Autodesk Fusion 360 part; units mm, degrees
sketch "Sketch1" plane through (0, 0, 0) normal (0, 0, 1) x (1, 0, 0)
  line L0 (97.7238, 100.1373) -> (197.7238, 100.1373)
  line L1 (197.7238, 100.1373) -> (197.7238, 30.1373)
  line L2 (197.7238, 30.1373) -> (97.7238, 30.1373)
  line L3 (97.7238, 30.1373) -> (97.7238, 100.1373)
  dimension "d1" = 70
  dimension "d2" = 100
extrude "Extrude1" add sketch "Sketch1" along normal blind 20
sketch "Sketch2" plane through (0, 0, 20) normal (0, 0, 1) x (-1, 0, 0)
  line L0 (-97.7238, -30.1373) -> (-197.7238, -30.1373)
  line L1 (-197.7238, -30.1373) -> (-197.7238, -100.1373)
  line L2 (-197.7238, -100.1373) -> (-97.7238, -100.1373)
  line L3 (-97.7238, -100.1373) -> (-97.7238, -30.1373)
  line L4 (-97.7238, -77.6373) -> (-127.7238, -77.6373)
  line L5 (-127.7238, -77.6373) -> (-127.7238, -52.6373)
  line L6 (-127.7238, -52.6373) -> (-97.7238, -52.6373)
  dimension "d5" = 22.5
  dimension "d6" = 22.5
  dimension "d7" = 25
  dimension "d8" = 30
  dimension "d9" = 25
extrude "Extrude2" cut sketch "Sketch2" against normal blind 27.453 contours L3 L4 L5 L6
sketch "Sketch3" plane through (0, 0, 20) normal (0, 0, 1) x (-1, 0, 0)
  line L0 (-127.7238, -52.6373) -> (-97.7238, -52.6373)
  line L1 (-97.7238, -52.6373) -> (-97.7238, -30.1373)
  line L2 (-97.7238, -30.1373) -> (-197.7238, -30.1373)
  line L3 (-197.7238, -30.1373) -> (-197.7238, -100.1373)
  line L4 (-197.7238, -100.1373) -> (-97.7238, -100.1373)
  line L5 (-97.7238, -100.1373) -> (-97.7238, -77.6373)
  line L6 (-97.7238, -77.6373) -> (-127.7238, -77.6373)
  line L7 (-127.7238, -77.6373) -> (-127.7238, -52.6373)
  line L8 (-97.7238, -52.6373) -> (-97.7238, -45.1373)
  line L9 (-97.7238, -77.6373) -> (-97.7238, -85.1373)
  line L10 (-147.7238, -30.1373) -> (-147.7238, -100.1373)
  line L11 (-97.7238, -85.1373) -> (-147.7238, -100.1373)
  line L12 (-97.7238, -45.1373) -> (-147.7238, -30.1373)
  dimension "d12" = 7.5
  dimension "d13" = 7.5
extrude "Extrude3" cut sketch "Sketch3" against normal blind 62.472 contours L1 L2 L12
extrude "Extrude4" cut sketch "Sketch3" against normal blind 73.462 contours L4 L5 L11
sketch "Sketch4" plane through (0, 30.1373, 0) normal (0, -1, 0) x (1, 0, 0)
  line L0 (147.7238, 20) -> (147.7238, 0)
  line L1 (147.7238, 0) -> (197.7238, 0)
  line L2 (197.7238, 0) -> (197.7238, 20)
  line L3 (197.7238, 20) -> (147.7238, 20)
  line L4 (197.7238, 20) -> (197.7238, 40)
  line L5 (197.7238, 40) -> (177.7238, 40)
  line L6 (177.7238, 40) -> (177.7238, 20)
  dimension "d18" = 20
  dimension "d19" = 20
extrude "Extrude5" add sketch "Sketch4" against normal blind 70 contours L3 L4 L5 L6
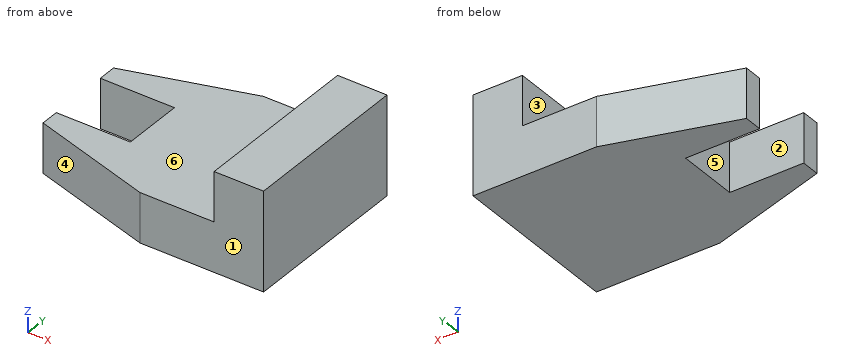
Work out the finished part from the listing and answer in its coordinate system (mm). Face numbers are marked on the shaded views. A direction names the side the tool comes from. Coordinates: 2 decimals unless noted, no trailing zeros. Loops run counter-clockwise (first coordinate to the right, second up) from the corner with the lowest first, then second, coordinate; pieces in that order, holes last.
1) Section A-A (z = 11.5) is taken. Give the vertices of the cut face in (x, y), plus the area to 3 significant figures.
Results:
outline: (97.72, 45.14) - (147.72, 30.14) - (197.72, 30.14) - (197.72, 100.14) - (147.72, 100.14) - (97.72, 85.14) - (97.72, 77.64) - (127.72, 77.64) - (127.72, 52.64) - (97.72, 52.64) - close
area: 5,500 mm2
2) Consider probe 1 along X at (y, z) = (43.5, 31); probe 2 along Z at (x, y) = (176, 73); probe 3 along X at (y, z) = (77.5, 18.5). Determine where each line is inside the solid, lowest interval first.
Results:
probe 1: x = 177.72 to 197.72
probe 2: z = 0 to 20
probe 3: x = 127.72 to 197.72
3) Flat-ended cylindrical pins translate along their axes: pin 1 (16 mm diameter, centred on x = 116, z = 9.5, fed in from +Y); pin 2 (8 mm diameter, centred on x = 139.5, z = 17.5, fed in from -Y); pin 3 (2 mm diameter, centred on x = 164, y = 48, fed in from +Z). Find the tip coordinate at first contact, or state that the pin passes through.
Results:
pin 1: stops at y = 93.02
pin 2: stops at y = 31.4
pin 3: stops at z = 20
4) For a pull along Y with two mould halves and no side action, classify the marked faces 4, 5 and 6 as +Y half, -Y half, draft (parallel to the pull), parting line (faces both ways), or undercut.
Results:
face 4: -Y half
face 5: undercut
face 6: draft
5) Section B-B (x = 106.5) is taken. Give the vertices of the cut face in (y, z), plus the area to 3 significant figures.
Results:
outline: (42.5, 0) - (52.64, 0) - (52.64, 20) - (42.5, 20) - close; (77.64, 0) - (87.77, 0) - (87.77, 20) - (77.64, 20) - close
area: 405 mm2
6) For the marked faces 1, 2 and 3, determine the directions among +Z, -Z, +X, -X, +Y, -Y from which every point of the face is accessible in a straight line to the end or side of a thin tool.
Results:
face 1: +Z, -Z, +X, -X, -Y
face 2: +Z, -Z, -X
face 3: +Z, -X, +Y, -Y
7) Section D-D (x = 175) is taken. Give the vertices of the cut face in (y, z), plus the area to 3 significant figures.
Results:
outline: (30.14, 0) - (100.14, 0) - (100.14, 20) - (30.14, 20) - close
area: 1,400 mm2
8) Section C-C (y = 69) is taken. Give the vertices of the cut face in (x, z), plus the area to 3 significant figures.
Results:
outline: (127.72, 0) - (197.72, 0) - (197.72, 40) - (177.72, 40) - (177.72, 20) - (127.72, 20) - close
area: 1,800 mm2
